Part model, mm, in its own coordinate system. A direction names the side the tool comes from. Round coordinates to 2 decimals unless told otherwise and drop trailing zeros. Order: outer loops, then holes, each group sorted by start corner. A loop starts at its lowest first (then second) coordinate and runs counter-clockwise, first axis right, second up. Notation, with made-up numbers: (-29.5, 42) -> (7.5, 42) arc R17 ccw to (7.5, 48) -> close; hole circle Ø9 at (-2, 32). An arc over 180 degrees is marked (long way). Return JSON: item names as keys, results as strings. Group by question number.
from build123d import *

# Parameters (mm, degrees)
SKETCH1_W           = 214
SKETCH1_H           = 114
BOSS_EXTRUDE1_DEPTH = 49.5
SKETCH2_R           = 2
CUT_EXTRUDE1_DEPTH  = 115
SKETCH4_R           = 30
SKETCH4_W           = 30
SKETCH4_H           = 74
CUT_EXTRUDE2_DEPTH  = 55


with BuildPart() as part:
    # Sketch1 → Boss-Extrude1 (new body)
    with BuildSketch(Plane(origin=(0, 0, 0), x_dir=(1, 0, 0), z_dir=(0, 1, 0))):
        Rectangle(SKETCH1_W, SKETCH1_H)
    extrude(amount=BOSS_EXTRUDE1_DEPTH)

    # Sketch2 → Cut-Extrude1 (cut, through all)
    with BuildSketch(Plane.XY.offset(57)):
        with Locations((-74.5, 38)):
            Circle(SKETCH2_R)
        with Locations((75.5, 38)):
            Circle(SKETCH2_R)
    extrude(amount=-CUT_EXTRUDE1_DEPTH, mode=Mode.SUBTRACT)

    # Sketch4 → Cut-Extrude2 (cut)
    with BuildSketch(Plane.XZ):
        with Locations((-62, -20)):
            Circle(SKETCH4_R)
        with Locations((62, 0)):
            Rectangle(SKETCH4_W, SKETCH4_H)
    extrude(amount=-CUT_EXTRUDE2_DEPTH, mode=Mode.SUBTRACT)


solid = part.part
(1) Probe L1, parallel to X at y = 38, z = -20.5; L2, parallel to X at y = 38, z = 16; L3, parallel to Y at x = -74.5, z = 35. List the from-to ranges inside material, lowest first. Write a range as [from, to].
(2) Mould opens along Y. For faces 1 (the flat face through (62, 24, -37)), 2 (the cylindrical face through (77.408, 38.601, 0.798)), 3 (the cylindrical face through (-76.498, 38.088, -51.549)), 4 (the flat face through (-1, 0, -1)) say: pulls with the +Y half, pulls with the -Y half, needs draft (parallel to the pull), parting line crosses it, or undercut.
(3) Saw through at D-D, the plane z = -34. List the corners of the cut face in (x, y), and give its area (3 significant figures).
(4) Saw through at A-A, the plane x = -62. List the corners of the cut face in (y, z).
(5) Saw through at B-B, the plane z = 23.5. List the corners of the cut face in (x, y), and give its area (3 significant figures).
(6) Tool access for faces 5 (the flat face through (107, 24, 1)), 6 (the flat face through (77, 44, -1)): list every direction of +Z, -Z, +X, -X, +Y, -Y with a clear straight run to the whole face (end or side of a thin tool).
(7) Saw through at C-C, the plane y = 45. List the corners of the cut face in (x, z).
Results are:
{
 "1": {"L1": "x = [-107, -92], [-32, 47], [77.5, 107]", "L2": "x = [-107, -76.5], [-72.5, 47], [77.5, 107]", "L3": "y = [0, 36], [40, 49.5]"},
 "2": {"face 1": "needs draft", "face 2": "undercut", "face 3": "undercut", "face 4": "pulls with the -Y half"},
 "3": {"outline": "(-107, 0) -> (-88.53, 0) -> (-88.53, 49.5) -> (-107, 49.5) -> close; (-35.47, 0) -> (47, 0) -> (47, 49.5) -> (-35.47, 49.5) -> close; (77, 0) -> (107, 0) -> (107, 49.5) -> (77, 49.5) -> (77, 39.32) arc R2 cw to (77, 36.68) -> close", "area": "6,480 mm^2"},
 "4": {"outline": "(0, -57) -> (49.5, -57) -> (49.5, -50) -> (0, -50) -> close; (0, 10) -> (49.5, 10) -> (49.5, 57) -> (0, 57) -> close"},
 "5": {"outline": "(-107, 0) -> (47, 0) -> (47, 49.5) -> (-107, 49.5) -> close; (77, 0) -> (107, 0) -> (107, 49.5) -> (77, 49.5) -> (77, 39.32) arc R2 cw to (77, 36.68) -> close; hole circle Ø4 at (-74.5, 38)", "area": "9,090 mm^2"},
 "6": {"face 5": "+Z, -Z, +X, +Y, -Y", "face 6": "+Y, -Y"},
 "7": {"outline": "(-107, -57) -> (107, -57) -> (107, 57) -> (-107, 57) -> close; hole circle Ø60 at (-62, -20); hole (47, -37) -> (77, -37) -> (77, 37) -> (47, 37) -> close"}
}
